The figure shows three views and two pictorial views of one solid part (mm, origin at its lowest corner). Answer the questions. Round coordinates to 2 decimals unless told otherwise and drop trailing zeros. Write each loop counter-clockwise with the first axis right and the second up, starting at its lowest first coordinate (ties: lowest second). Pieces come first, ordered by that corner, then holes. Notation, with made-up numbers: M 17,-14 L 24,-14 A24 ccw 24,4 Z; hole C 31.5,64 d5. An arc over 180 degrees is marked long. Answer in a Markdown table with one row per item.
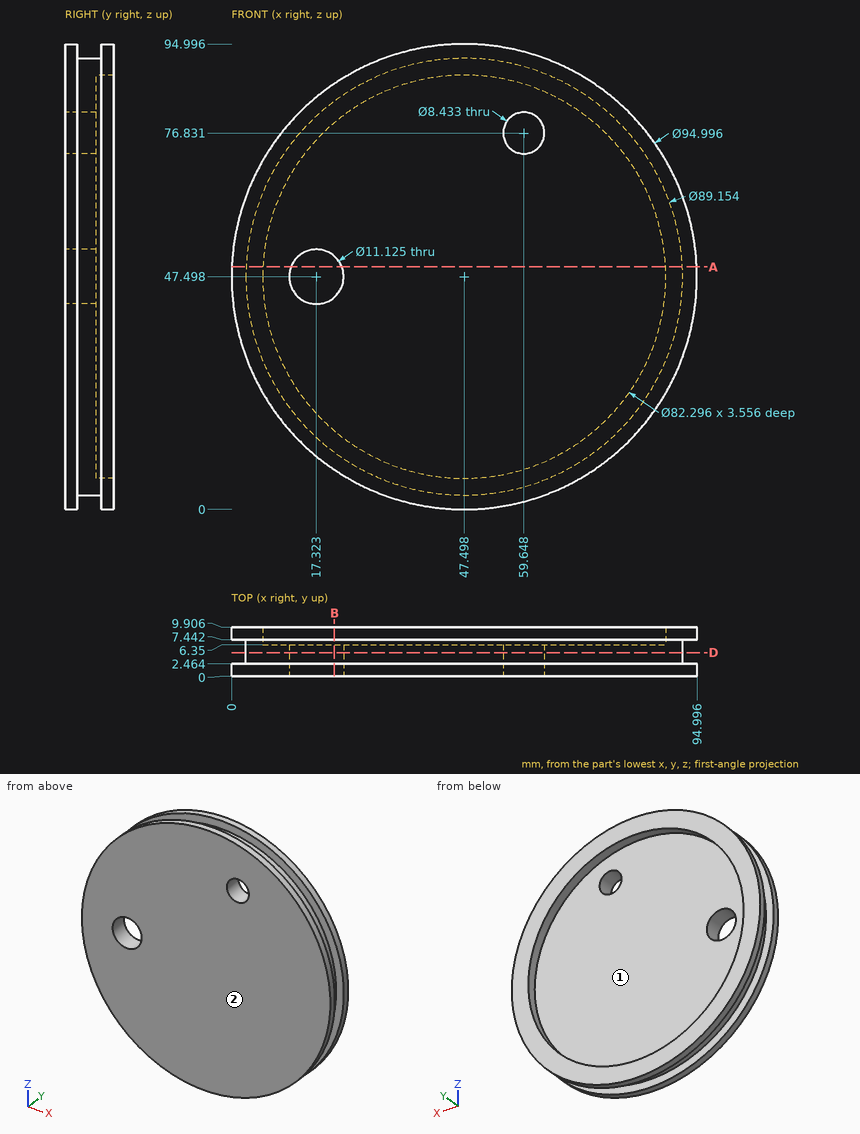
1. The part is cut by section D-D (y = 4.75). Determine the outline of the cut face in (x, z) (1 decimal), plus the area to 3 significant figures.
Calculated:
| item | result |
|---|---|
| outline | C 47.5,47.5 d89.2; hole C 17.3,47.5 d11.1; hole C 59.6,76.8 d8.4 |
| area | 6,090 mm² |
2. The part is cut by section B-B (x = 21). Determine the outline of the cut face in (y, z).
Calculated:
| item | result |
|---|---|
| outline | M 0,8.08 L 2.46,8.08 L 2.46,11.65 L 7.44,11.65 L 7.44,8.08 L 9.91,8.08 L 9.91,16.02 L 6.35,16.02 L 6.35,43.32 L 0,43.32 Z; M 0,51.67 L 6.35,51.67 L 6.35,78.98 L 9.91,78.98 L 9.91,86.92 L 7.44,86.92 L 7.44,83.34 L 2.46,83.34 L 2.46,86.92 L 0,86.92 Z |
3. Consider line 1 along Y through (x, z) = (26, 7.5); line 2 along Y through (x, z) = (47, 22); line 3 along Z through (x, y) = (59.5, 7). Determine where each line is inside the solid, lowest interval first. Write a range as from..to.
Calculated:
| item | result |
|---|---|
| line 1 | y = 0..2.46, 7.44..9.91 |
| line 2 | y = 0..6.35 |
| line 3 | z = 4.57..8.14, 86.86..90.43 |
4. Given pin 1 (10 mm diameter, centred on x = 17.32, z = 47.5, fed in from -Y); pin 2 (13.5 mm diameter, centred on x = 59.65, z = 76.83, fed in from +Y); pin 3 (1.5 mm diameter, centred on y = 3.5, z = 42.5, fed in from -X), each flat-ended and moving along its own axis, determine where each tip first touches the part or whether it passes through.
Calculated:
| item | result |
|---|---|
| pin 1 | passes through |
| pin 2 | stops at y = 6.35 |
| pin 3 | stops at x = 3.12 |
5. Determine the mould class of the marked faces 1 and 2 for opening direction Z: released by +Z, released by -Z, zero draft, split by the parting line, or undercut.
Calculated:
| item | result |
|---|---|
| face 1 | undercut |
| face 2 | zero draft |
6. The part is cut by section A-A (z = 49.5). Determine the outline of the cut face in (x, y).
Calculated:
| item | result |
|---|---|
| outline | M 0.04,0 L 12.13,0 L 12.13,6.35 L 6.4,6.35 L 6.4,9.91 L 0.04,9.91 L 0.04,7.44 L 2.97,7.44 L 2.97,2.46 L 0.04,2.46 Z; M 22.51,0 L 94.95,0 L 94.95,2.46 L 92.03,2.46 L 92.03,7.44 L 94.95,7.44 L 94.95,9.91 L 88.6,9.91 L 88.6,6.35 L 22.51,6.35 Z |
